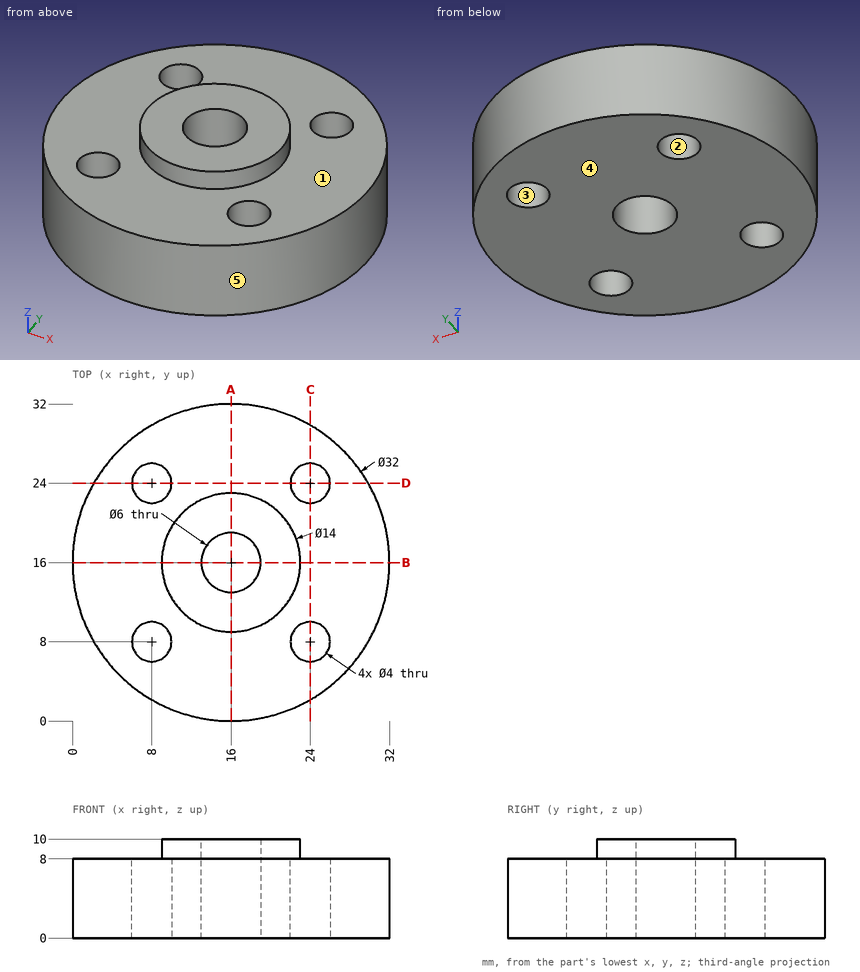
Source: three-view drawing plus pictorial views. Frame: mm from the lowest corner of the part. A direction names the side the tool comes from. Give positions to 0.01 mm unless a question says otherwise; leave off trailing zeros. Loops run counter-clockwise (first coordinate to the right, second up) from the corner with the lowest first, then second, coordinate; pieces in that order, holes last. Notation, with made-up numbers: (-4.5, -3) -> (51.5, -3) arc R20 ccw to (51.5, 7) -> close; hole circle Ø10 at (27.5, 33). An arc over 180 degrees is marked (long way). Put each result on its own line as item: value. Start each with the question number.
1) Draft query along X for the marked faces 3, 4 and 5. Return one class per face: released by +X, released by -X, zero draft, split by the parting line, or undercut.
2) Contact query for flat-ended pins moving along their axis: P1, Ø1.5, axis at x = 10.5, z = 5.5, coming from the +Y side; P2, Ø1.5, axis at y = 18.5, z = 2.5, coming from the +X side; P3, Ø2.5, axis at x = 24, y = 24, coming from the +Z side; P4, Ø3, axis at y = 28.5, z = 5, coming from the -X side. Output: stop coordinate, or through.
3) Cut plane C-C (x = 24). Return loops of the section in (y, z).
4) Material intervals for probe 1 along Y at (x, z) = (16, 3.75); probe 2 along X at (y, z) = (8.5, 3.5); probe 3 along X at (y, z) = (9.5, 0.5), sorted ascending.
5) Reachability of the marked faces 1 and 2 from +Z, -Z, +X, -X, +Y, -Y: full face, straight path, thin tool, end or side. Return the list, or none.
6) Cut plane A-A (x = 16). Return loops of the section in (y, z), then the cut area to 3 significant figures.
Results are:
1. face 3: undercut
1. face 4: zero draft
1. face 5: split by the parting line
2. P1: stops at y = 31.28
2. P2: stops at x = 31.9
2. P3: passes through
2. P4: stops at x = 4.38
3. outline: (2.14, 0) -> (6, 0) -> (6, 8) -> (2.14, 8) -> close; (10, 0) -> (22, 0) -> (22, 8) -> (10, 8) -> close; (26, 0) -> (29.86, 0) -> (29.86, 8) -> (26, 8) -> close
4. probe 1: y = 0 to 13, 19 to 32
4. probe 2: x = 1.87 to 6.06, 9.94 to 22.06, 25.94 to 30.13
4. probe 3: x = 1.38 to 6.68, 9.32 to 22.68, 25.32 to 30.62
5. face 1: +Z
5. face 2: +Z, -Z
6. outline: (0, 0) -> (13, 0) -> (13, 10) -> (9, 10) -> (9, 8) -> (0, 8) -> close; (19, 0) -> (32, 0) -> (32, 8) -> (23, 8) -> (23, 10) -> (19, 10) -> close
6. area: 224 mm2
